from build123d import *

# Parameters (mm, degrees)
SCHIZZO1_W                               = 96
SCHIZZO1_H                               = 76
ESTRUSIONE_ESTRUSIONE1_DEPTH             = 1
TAGLIO_ESTRUSIONE1_DEPTH                 = 62.253571324
TAGLIO_ESTRUSIONE1_DEPTH_BACK            = 62.253571324
SCHIZZO2_R                               = 15
TAGLIO_ESTRUSIONE2_DEPTH                 = 62.253571324
RACCORDO1_R                              = 4
SPECCHIA1_START                          = -1
SPECCHIA1_DEPTH                          = 2
FORO_SVASATO_PER_VITE_M2_5_1_D           = 2.9
FORO_SVASATO_PER_VITE_M2_5_1_DEPTH       = 8.25
FORO_SVASATO_PER_VITE_M2_5_1_CSINK_D     = 5.5
FORO_SVASATO_PER_VITE_M2_5_1_CSINK_ANGLE = 90
FORO_SVASATO_PER_VITE_M2_5_1_TIP         = 0.871247898


# Read off the part's stored shape, not the designer's step: Specchia1
with BuildPart() as part:
    # Schizzo1 → Estrusione-Estrusione1 (new, symmetric)
    with BuildSketch(Plane(origin=(0, 0, 0), x_dir=(1, 0, 0), z_dir=(0, 1, 0))):
        Rectangle(SCHIZZO1_W, SCHIZZO1_H)
    extrude(amount=ESTRUSIONE_ESTRUSIONE1_DEPTH, both=True)

    # Schizzo2 → Taglio-Estrusione1 (cut, two sides: drawn at the far end of the back side and taken through both)
    with BuildSketch(Plane(origin=(0, 1, 0), x_dir=(1, 0, 0), z_dir=(0, 1, 0)).offset(-TAGLIO_ESTRUSIONE1_DEPTH_BACK)):
        with Locations(Location((0, 0, 0), (0, 0, 270))):
            Circle(SCHIZZO2_R)
    extrude(amount=TAGLIO_ESTRUSIONE1_DEPTH + TAGLIO_ESTRUSIONE1_DEPTH_BACK, mode=Mode.SUBTRACT)

    # Schizzo3 → Taglio-Estrusione2 (cut, through all)
    with BuildSketch(Plane(origin=(0, 1, 0), x_dir=(1, 0, 0), z_dir=(0, 1, 0))):
        with BuildLine():
            Line((-2.5, 30), (-2.5, 19.843134833))
            ThreePointArc((-2.5, 19.843134833), (-14.142135624, 14.142135624), (-19.843134833, 2.5))
            Line((-19.843134833, 2.5), (-40, 2.5))
            Line((-40, 2.5), (-40, 30))
            Line((-40, 30), (-2.5, 30))
        make_face()
    extrude(amount=-TAGLIO_ESTRUSIONE2_DEPTH, mode=Mode.SUBTRACT)

    # Raccordo1
    raccordo1_edges = [part.edges().sort_by_distance(p)[0] for p in [
        (-40, 0, -2.5),
        (-40, 0, -30),
        (-2.5, 0, -30),
        (-2.5, 0, -19.843134833),
        (-19.843134833, 0, -2.5),
    ]]
    fillet(raccordo1_edges, radius=RACCORDO1_R)

    # Specchia1 outline → Specchia1 (cut)
    with BuildSketch(Plane(origin=(0, 0, 0), x_dir=(1, 0, 0), z_dir=(0, 1, 0)).offset(SPECCHIA1_START)):
        with BuildLine():
            Line((-40, -6.5), (-40, -26))
            ThreePointArc((-40, -26), (-38.828427125, -28.828427125), (-36, -30))
            Line((-36, -30), (-6.5, -30))
            ThreePointArc((-6.5, -30), (-3.671572875, -28.828427125), (-2.5, -26))
            Line((-2.5, -26), (-2.5, -23.103030104))
            ThreePointArc((-2.5, -23.103030104), (-3.311478922, -20.687800647), (-5.416666667, -19.252525087))
            ThreePointArc((-5.416666667, -19.252525087), (-14.142135624, -14.142135624), (-19.252525087, -5.416666667))
            ThreePointArc((-19.252525087, -5.416666667), (-20.687800647, -3.311478922), (-23.103030104, -2.5))
            Line((-23.103030104, -2.5), (-36, -2.5))
            ThreePointArc((-36, -2.5), (-38.828427125, -3.671572875), (-40, -6.5))
        make_face()
        with BuildLine():
            Line((36, 30), (6.5, 30))
            ThreePointArc((6.5, 30), (3.671572875, 28.828427125), (2.5, 26))
            Line((2.5, 26), (2.5, 23.103030104))
            ThreePointArc((2.5, 23.103030104), (3.311478922, 20.687800647), (5.416666667, 19.252525087))
            ThreePointArc((5.416666667, 19.252525087), (14.142135624, 14.142135624), (19.252525087, 5.416666667))
            ThreePointArc((19.252525087, 5.416666667), (20.687800647, 3.311478922), (23.103030104, 2.5))
            Line((23.103030104, 2.5), (36, 2.5))
            ThreePointArc((36, 2.5), (38.828427125, 3.671572875), (40, 6.5))
            Line((40, 6.5), (40, 26))
            ThreePointArc((40, 26), (38.828427125, 28.828427125), (36, 30))
        make_face()
        with BuildLine():
            ThreePointArc((19.252525087, -5.416666667), (14.142135624, -14.142135624), (5.416666667, -19.252525087))
            ThreePointArc((5.416666667, -19.252525087), (3.311478922, -20.687800647), (2.5, -23.103030104))
            Line((2.5, -23.103030104), (2.5, -26))
            ThreePointArc((2.5, -26), (3.671572875, -28.828427125), (6.5, -30))
            Line((6.5, -30), (36, -30))
            ThreePointArc((36, -30), (38.828427125, -28.828427125), (40, -26))
            Line((40, -26), (40, -6.5))
            ThreePointArc((40, -6.5), (38.828427125, -3.671572875), (36, -2.5))
            Line((36, -2.5), (23.103030104, -2.5))
            ThreePointArc((23.103030104, -2.5), (20.687800647, -3.311478922), (19.252525087, -5.416666667))
        make_face()
    extrude(amount=SPECCHIA1_DEPTH, mode=Mode.SUBTRACT)

    # Foro svasato per Vite M2.5-1
    with Locations(Plane(origin=(0, 1, 0), x_dir=(1, 0, 0), z_dir=(0, 1, 0))):
        with Locations((-25, 34), (25, 34), (25, -34), (-25, -34)):
            CounterSinkHole(FORO_SVASATO_PER_VITE_M2_5_1_D / 2, FORO_SVASATO_PER_VITE_M2_5_1_CSINK_D / 2, depth=FORO_SVASATO_PER_VITE_M2_5_1_DEPTH, counter_sink_angle=FORO_SVASATO_PER_VITE_M2_5_1_CSINK_ANGLE)
            with Locations((0, 0, -(FORO_SVASATO_PER_VITE_M2_5_1_DEPTH + FORO_SVASATO_PER_VITE_M2_5_1_TIP / 2))):  # 118° drill point
                Cone(0, FORO_SVASATO_PER_VITE_M2_5_1_D / 2, FORO_SVASATO_PER_VITE_M2_5_1_TIP, mode=Mode.SUBTRACT)


solid = part.part
Could you check a few things on this model? Use its own coordinates, in mm. Give positions to 0.01 mm unless a question says otherwise; leave off trailing zeros. Loops run counter-clockwise (first coordinate to the right, second up) from the corner with the lowest first, then second, coordinate; pieces in that order, holes last. Notation, with made-up numbers: (8.5, 77) -> (52.5, 77) arc R15 cw to (52.5, 92) -> close; hole circle Ø3 at (4, 53.25). An arc over 180 degrees is marked (long way). Return JSON: item names as keys, results as strings.
Item 1: If we section it at B-B on z = 0: List the corners of the cut face in (x, y) for me, plus the area to 3 significant figures.
Geometry results:
{"outline": "(-48, -1) -> (-15, -1) -> (-15, 1) -> (-48, 1) -> close; (15, -1) -> (48, -1) -> (48, 1) -> (15, 1) -> close", "area": "132 mm²"}
Item 2: If we section it at D-D on z = -12.5: List the corners of the cut face in (x, y) for me, plus the area to 3 significant figures.
Geometry results:
{"outline": "(-48, -1) -> (-40, -1) -> (-40, 1) -> (-48, 1) -> close; (-15.61, -1) -> (-8.29, -1) -> (-8.29, 1) -> (-15.61, 1) -> close; (8.29, -1) -> (15.61, -1) -> (15.61, 1) -> (8.29, 1) -> close; (40, -1) -> (48, -1) -> (48, 1) -> (40, 1) -> close", "area": "61.3 mm²"}
Item 3: If we section it at C-C on x = -35: List the corners of the cut face in (y, z) for me.
Geometry results:
{"outline": "(-1, -38) -> (1, -38) -> (1, -30) -> (-1, -30) -> close; (-1, -2.5) -> (1, -2.5) -> (1, 2.5) -> (-1, 2.5) -> close; (-1, 30) -> (1, 30) -> (1, 38) -> (-1, 38) -> close"}
Item 4: If we section it at A-A on x = 0: List the corners of the cut face in (y, z) for me, plus the area to 3 significant figures.
Geometry results:
{"outline": "(-1, -38) -> (1, -38) -> (1, -15) -> (-1, -15) -> close; (-1, 15) -> (1, 15) -> (1, 38) -> (-1, 38) -> close", "area": "92.0 mm²"}
Item 5: I need wall thicknesses on L1, parallel to Z at x = 25, y = -0.65; L2, parallel to X at y = -0.8, z = -34; L3, parallel to Z at x = 0, y = -0.55. Which ranges of each line are inside material? Lowest first, please. Write a range as from..to.
Geometry results:
{"L1": "z = -38..-35.45, -32.55..-30, -2.5..2.5, 30..32.55, 35.45..38", "L2": "x = -48..-26.45, -23.55..23.55, 26.45..48", "L3": "z = -38..-15, 15..38"}
